The model under review builds one solid part; all positions refer to its coordinate system, in mm. Give positions to 0.01 mm unless a question says otherwise; leave off trailing zeros. Loops run counter-clockwise (first coordinate to the right, second up) from the corner with the lowest first, then second, coordinate; pieces in that order, holes last. Notation, with made-up numbers: (4.5, 27) - (15.5, 27) arc R9 ccw to (15.5, 40) - close; hole circle Ø9 at (34, 42.5). An arc over 180 degrees is marked (long way). Return JSON: item names as keys, results as strings. Group by question number.
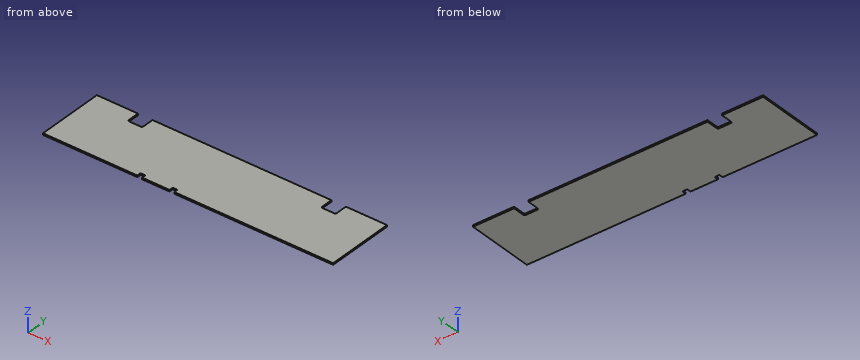
from build123d import *

# Parameters (mm, degrees)
BOSS_EXTRUDE1_DEPTH = 6.35
FILLET1_R           = 6.35
SKETCH2_W           = 19.05
SKETCH2_H           = 15.875
CUT_EXTRUDE1_DEPTH  = 7.35
FILLET2_R           = 3.175


with BuildPart() as part:
    # Sketch1 → Boss-Extrude1 (new body)
    with BuildSketch(Plane.XY):
        Polygon((0, 0), (0, 266.7), (161.925, 266.7), (161.925, 215.9), (219.075, 215.9), (219.075, 266.7), (923.925, 266.7), (923.925, 215.9), (981.075, 215.9), (981.075, 266.7), (1143, 266.7), (1143, 0), align=None)
    extrude(amount=BOSS_EXTRUDE1_DEPTH)

    # Fillet1
    fillet1_edges = [part.edges().sort_by_distance(p)[0] for p in [
        (161.925, 215.9, 3.175),
        (219.075, 215.9, 3.175),
        (923.925, 215.9, 3.175),
        (981.075, 215.9, 3.175),
    ]]
    fillet(fillet1_edges, radius=FILLET1_R)

    # Sketch2 → Cut-Extrude1 (cut, through all)
    with BuildSketch(Plane.XY.offset(6.35)):
        with Locations((381, 7.9375)):
            Rectangle(SKETCH2_W, SKETCH2_H)
        with Locations((508, 7.9375)):
            Rectangle(SKETCH2_W, SKETCH2_H)
    extrude(amount=-CUT_EXTRUDE1_DEPTH, mode=Mode.SUBTRACT)

    # Fillet2
    fillet2_edges = [part.edges().sort_by_distance(p)[0] for p in [
        (371.475, 15.875, 3.175),
        (390.525, 15.875, 3.175),
        (498.475, 15.875, 3.175),
        (517.525, 15.875, 3.175),
    ]]
    fillet(fillet2_edges, radius=FILLET2_R)


solid = part.part
Item 1: For L1, parallel to X at y = 232, z = 3.5 (3 decimals); L2, parallel to Y at x = 188.5, z = 2, list the stretches that pass through material, from the lowest coordinate up. Write a range as from..to.
Item 2: Take a section at A-A (y = 232). State the section outline as (x, z) points (3 decimals).
Item 3: Take a section at B-B (z = 4.75). State the section outline as (x, y) points (3 decimals), then the cut area to 3 significant figures.
Item 4: Take a section at C-C (x = 190.5). State the section outline as (y, z) points, then the cut area to 3 significant figures.
Check sheet entries:
{
 "1": {"L1": "x = 0..161.925, 219.075..923.925, 981.075..1143", "L2": "y = 0..215.9"},
 "2": {"outline": "(0, 0) - (161.925, 0) - (161.925, 6.35) - (0, 6.35) - close; (219.075, 0) - (923.925, 0) - (923.925, 6.35) - (219.075, 6.35) - close; (981.075, 0) - (1143, 0) - (1143, 6.35) - (981.075, 6.35) - close"},
 "3": {"outline": "(0, 0) - (371.475, 0) - (371.475, 12.7) arc R3.175 cw to (374.65, 15.875) - (387.35, 15.875) arc R3.175 cw to (390.525, 12.7) - (390.525, 0) - (498.475, 0) - (498.475, 12.7) arc R3.175 cw to (501.65, 15.875) - (514.35, 15.875) arc R3.175 cw to (517.525, 12.7) - (517.525, 0) - (1143, 0) - (1143, 266.7) - (981.075, 266.7) - (981.075, 222.25) arc R6.35 cw to (974.725, 215.9) - (930.275, 215.9) arc R6.35 cw to (923.925, 222.25) - (923.925, 266.7) - (219.075, 266.7) - (219.075, 222.25) arc R6.35 cw to (212.725, 215.9) - (168.275, 215.9) arc R6.35 cw to (161.925, 222.25) - (161.925, 266.7) - (0, 266.7) - close", "area": "298,000 mm^2"},
 "4": {"outline": "(0, 0) - (215.9, 0) - (215.9, 6.35) - (0, 6.35) - close", "area": "1,370 mm^2"}
}
